Read the model definition and answer for the solid it produces. Units are mm, in the model's axes. Face numbers are marked on the shaded views. Round coordinates to 2 decimals unless told otherwise and drop trailing zeros. Order: outer loops, then holes, each group sorted by start corner. A loop starts at its lowest first (then second) coordinate and runs counter-clockwise, first axis right, second up. Notation, with made-up numbers: (74, -23) -> (123, -23) arc R17 ccw to (123, 3) -> close; hole circle Ø7 at (88.25, 45.5). An arc over 180 degrees is marked (long way). Use a Markdown table: item, result. Add a question column.
1. Section B-B, the plane z = 6 is taken. Give the vertices of the cut face in (x, y).
2. Section C-C, the plane y = 1.3 is taken. Give the vertices of the cut face in (x, z), then the cut area to 3 significant figures.
3. Given pin 1 (6 mm diameter, centred on x = -3.5, z = 1, fed in from +Y), flat-ended and moving along its own axis, determine where the tip first touches the part or whether it passes through.
4. Consider L1, parallel to X at y = 4.1, z = 2; L2, parallel to Y at x = -6.25, z = 1.25; L3, parallel to Z at x = 2.25, y = 0.7. Determine where each line is inside the solid, lowest interval first. Write a range as [from, to].
5. Section A-A, the plane x = -3.5 is taken. Give the vertices of the cut face in (y, z).
6. The mould has two halves that part along X. Classify the marked faces 1, 2, 3 and 4: +X half, -X half, draft (parallel to the pull), parting line (faces both ways), or undercut.
7. Section D-D, the plane x = 2.25 is taken. Give the vertices of the cut face in (y, z), then the cut area to 3 significant figures.
```python
from build123d import *

# Parameters (mm, degrees)
BOSS_EXTRUDE1_DEPTH = 3
BOSS_EXTRUDE2_DEPTH = 5


with BuildPart() as part:
    # Sketch1 → Boss-Extrude1 (new body)
    with BuildSketch(Plane(origin=(0, 0, 0), x_dir=(1, 0, 0), z_dir=(0, 1, 0))):
        with BuildLine():
            ThreePointArc((-10, -7.5), (-8.619130411, -9.053208876), (-7, -10.356157589))
            Line((-7, -10.356157589), (-7, 10.356157589))
            ThreePointArc((-7, 10.356157589), (-8.619130411, 9.053208876), (-10, 7.5))
            Line((-10, 7.5), (-10, -7.5))
        make_face()
        with BuildLine():
            ThreePointArc((-7, -10.356157589), (-3.66046651, -11.952028486), (0, -12.5))
            Line((0, -12.5), (0, -4))
            ThreePointArc((0, -4), (-4, 0), (0, 4))
            Line((0, 4), (0, 12.5))
            ThreePointArc((0, 12.5), (-3.66046651, 11.952028486), (-7, 10.356157589))
            Line((-7, 10.356157589), (-7, -10.356157589))
        make_face()
        with BuildLine():
            Line((0, -4), (0, -12.5))
            ThreePointArc((0, -12.5), (3.66046651, -11.952028486), (7, -10.356157589))
            Line((7, -10.356157589), (7, 10.356157589))
            ThreePointArc((7, 10.356157589), (3.66046651, 11.952028486), (0, 12.5))
            Line((0, 12.5), (0, 4))
            ThreePointArc((0, 4), (2.828427125, 2.828427125), (4, 0))
            ThreePointArc((4, 0), (2.828427125, -2.828427125), (0, -4))
        make_face()
        with BuildLine():
            Line((7, 10.356157589), (7, -10.356157589))
            ThreePointArc((7, -10.356157589), (8.619130411, -9.053208876), (10, -7.5))
            Line((10, -7.5), (10, 7.5))
            ThreePointArc((10, 7.5), (8.619130411, 9.053208876), (7, 10.356157589))
        make_face()
    extrude(amount=BOSS_EXTRUDE1_DEPTH)

    # Sketch1_3 → Boss-Extrude2 (add)
    with BuildSketch(Plane(origin=(0, 0, 0), x_dir=(1, 0, 0), z_dir=(0, 1, 0))):
        with BuildLine():
            Line((-10, 7.5), (-10, -7.5))
            ThreePointArc((-10, -7.5), (-8.619130411, -9.053208876), (-7, -10.356157589))
            Line((-7, -10.356157589), (-7, 10.356157589))
            ThreePointArc((-7, 10.356157589), (-8.619130411, 9.053208876), (-10, 7.5))
        make_face()
        with BuildLine():
            Line((7, 10.356157589), (7, -10.356157589))
            ThreePointArc((7, -10.356157589), (8.619130411, -9.053208876), (10, -7.5))
            Line((10, -7.5), (10, 7.5))
            ThreePointArc((10, 7.5), (8.619130411, 9.053208876), (7, 10.356157589))
        make_face()
    extrude(amount=BOSS_EXTRUDE2_DEPTH)


solid = part.part
```
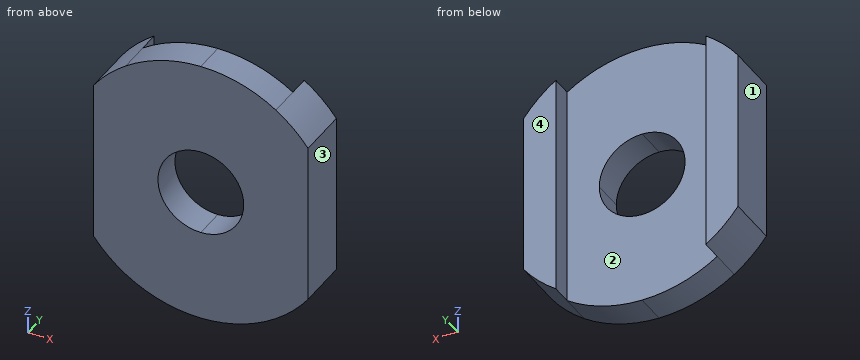
Verdict:
| question | item | result |
|---|---|---|
| 1 | outline | (-10, 0) -> (10, 0) -> (10, 5) -> (7, 5) -> (7, 3) -> (-7, 3) -> (-7, 5) -> (-10, 5) -> close |
| 2 | outline | (-10, -7.5) arc R12.5 ccw to (10, -7.5) -> (10, 7.5) arc R12.5 ccw to (-10, 7.5) -> close; hole circle Ø8 at (0, 0) |
| 2 | area | 390 mm2 |
| 3 | pin 1 | stops at y = 3 |
| 4 | L1 | x = [-10, -7], [7, 10] |
| 4 | L2 | y = [0, 3] |
| 4 | L3 | z = [-12.3, -3.31], [3.31, 12.3] |
| 5 | outline | (0, -12) -> (3, -12) -> (3, -1.94) -> (0, -1.94) -> close; (0, 1.94) -> (3, 1.94) -> (3, 12) -> (0, 12) -> close |
| 6 | face 1 | -X half |
| 6 | face 2 | undercut |
| 6 | face 3 | +X half |
| 6 | face 4 | draft |
| 7 | outline | (0, -12.3) -> (3, -12.3) -> (3, -3.31) -> (0, -3.31) -> close; (0, 3.31) -> (3, 3.31) -> (3, 12.3) -> (0, 12.3) -> close |
| 7 | area | 53.9 mm2 |
